```python
from build123d import *

# Parameters (mm, degrees)
SKETCH1_W           = 25.4
SKETCH1_H           = 25.4
BOSS_EXTRUDE1_DEPTH = 203.2
SKETCH2_R           = 3.175
CUT_EXTRUDE1_DEPTH  = 207.350575478
SKETCH3_W           = 12.7
SKETCH3_H           = 12.7
CUT_EXTRUDE2_DEPTH  = 207.350575478


with BuildPart() as part:
    # Sketch1 → Boss-Extrude1 (new body)
    with BuildSketch(Plane.XY):
        with Locations((-12.7, 12.7)):
            Rectangle(SKETCH1_W, SKETCH1_H)
    extrude(amount=BOSS_EXTRUDE1_DEPTH)

    # Sketch2 → Cut-Extrude1 (cut, through all)
    with BuildSketch(Plane(origin=(0, 0, 0), x_dir=(0, 0, -1), z_dir=(1, 0, 0))):
        with Locations(Location((-63.5, 12.7, 0), (0, 0, 90))):
            Circle(SKETCH2_R)
    extrude(amount=-CUT_EXTRUDE1_DEPTH, mode=Mode.SUBTRACT)

    # Sketch3 → Cut-Extrude2 (cut, through all)
    with BuildSketch(Plane(origin=(0, 0, 0), x_dir=(-1, 0, 0), z_dir=(0, 0, -1))):
        with Locations((12.7, 12.7)):
            Rectangle(SKETCH3_W, SKETCH3_H)
    extrude(amount=-CUT_EXTRUDE2_DEPTH, mode=Mode.SUBTRACT)


solid = part.part
```
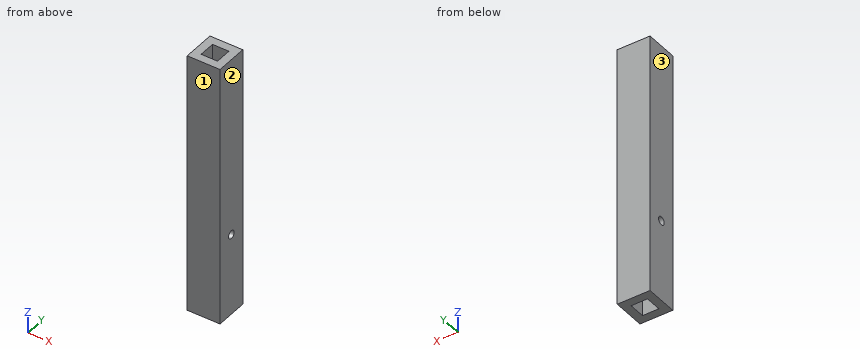
The listing builds one solid part. Answer for the finished solid, in the listing's coordinates (mm). Face numbers are marked on the shaded views. Coordinates: 2 decimals unless noted, no trailing zeros. Loops run counter-clockwise (first coordinate to the right, second up) from the corner with the lowest first, then second, coordinate; pieces in that order, holes last. Notation, with made-up numbers: (67, 4) -> (94, 4) arc R17 ccw to (94, 27) -> close; hole circle Ø6 at (5, -4.75). An arc over 180 degrees is marked (long way). Return JSON: item names as keys, results as strings. Group by question number.
(1) A cutting plane is placed at C-C on y = 12.7. Write down the section's boundary in (x, z) (3 decimals), and give its area (3 significant figures).
(2) A cutting plane is placed at D-D on z = 123.5. Write down the section's boundary in (x, y).
(3) Find the intervals of material crossed by probe 1 along Y at (x, z) = (-16.25, 171); probe 2 along Z at (x, y) = (-23.5, 12.7) (3 decimals); probe 3 along X at (y, z) = (9, 78), in increasing order. Write a range as from..to.
(4) A cutting plane is placed at A-A on x = -11.5. Write down the section's boundary in (y, z), and give its area (3 significant figures).
(5) Determine the mould class of the marked faces 1, 2 and 3 for opening direction X: released by +X, released by -X, zero draft, split by the parting line, or undercut.
(6) A cutting plane is placed at B-B on z = 63.5. Write down the section's boundary in (x, y) (3 decimals).
The answers:
{
 "1": {"outline": "(-25.4, 0) -> (-19.05, 0) -> (-19.05, 60.325) -> (-25.4, 60.325) -> close; (-25.4, 66.675) -> (-19.05, 66.675) -> (-19.05, 203.2) -> (-25.4, 203.2) -> close; (-6.35, 0) -> (0, 0) -> (0, 60.325) -> (-6.35, 60.325) -> close; (-6.35, 66.675) -> (0, 66.675) -> (0, 203.2) -> (-6.35, 203.2) -> close", "area": "2,500 mm^2"},
 "2": {"outline": "(-25.4, 0) -> (0, 0) -> (0, 25.4) -> (-25.4, 25.4) -> close; hole (-19.05, 6.35) -> (-6.35, 6.35) -> (-6.35, 19.05) -> (-19.05, 19.05) -> close"},
 "3": {"probe 1": "y = 0..6.35, 19.05..25.4", "probe 2": "z = 0..60.325, 66.675..203.2", "probe 3": "x = -25.4..-19.05, -6.35..0"},
 "4": {"outline": "(0, 0) -> (6.35, 0) -> (6.35, 203.2) -> (0, 203.2) -> close; (19.05, 0) -> (25.4, 0) -> (25.4, 203.2) -> (19.05, 203.2) -> close", "area": "2,580 mm^2"},
 "5": {"face 1": "zero draft", "face 2": "released by +X", "face 3": "released by -X"},
 "6": {"outline": "(-25.4, 0) -> (0, 0) -> (0, 9.525) -> (-6.35, 9.525) -> (-6.35, 6.35) -> (-19.05, 6.35) -> (-19.05, 9.525) -> (-25.4, 9.525) -> close; (-25.4, 15.875) -> (-19.05, 15.875) -> (-19.05, 19.05) -> (-6.35, 19.05) -> (-6.35, 15.875) -> (0, 15.875) -> (0, 25.4) -> (-25.4, 25.4) -> close"}
}
